Check sheet for the modelled part. Datum: model origin and axes. Units: mm. A direction names the side the tool comes from. Coordinates: 2 decimals unless noted, no trailing zeros. Loops run counter-clockwise (first coordinate to the right, second up) from the corner with the lowest first, then second, coordinate; pieces in that order, holes last.
```python
from build123d import *

# Parameters (mm, degrees)
ESQUISSE1_W             = 105
ESQUISSE1_H             = 30
BOSS_EXTRU_1_DEPTH      = 25
ESQUISSE2_W             = 2
ESQUISSE2_H             = 25
ENL_V_MAT_EXTRU_1_DEPTH = 24
CONG_3_R                = 12
CONG_4_R                = 12
ESQUISSE3_W             = 84
ESQUISSE3_H             = 24
ENL_V_MAT_EXTRU_2_DEPTH = 20
CONG_5_R                = 2
CONG_6_R                = 2
CONG_7_R                = 2


with BuildPart() as part:
    # Esquisse1 → Boss.-Extru.1 (new body)
    with BuildSketch(Plane.XY):
        with Locations((10.65403423, 34.547677262)):
            Rectangle(ESQUISSE1_W, ESQUISSE1_H)
    extrude(amount=BOSS_EXTRU_1_DEPTH)

    # Esquisse2 → Enlèv. mat.-Extru.1 (cut)
    with BuildSketch(Plane.XY.offset(25)):
        with Locations((-34.34596577, 35.047677262)):
            Rectangle(ESQUISSE2_W, ESQUISSE2_H)
        with Locations((55.65403423, 35.047677262)):
            Rectangle(ESQUISSE2_W, ESQUISSE2_H)
    extrude(amount=-ENL_V_MAT_EXTRU_1_DEPTH, mode=Mode.SUBTRACT)

    # Congé3
    cong_3_edges = [part.edges().sort_by_distance(p)[0] for p in [
        (55.65403423, 47.547677262, 1),
        (55.65403423, 22.547677262, 1),
    ]]
    fillet(cong_3_edges, radius=CONG_3_R)

    # Congé4
    cong_4_edges = [part.edges().sort_by_distance(p)[0] for p in [
        (-34.34596577, 47.547677262, 1),
        (-34.34596577, 22.547677262, 1),
    ]]
    fillet(cong_4_edges, radius=CONG_4_R)

    # Esquisse3 → Enlèv. mat.-Extru.2 (cut)
    with BuildSketch(Plane.XY.offset(25)):
        with Locations((10.65403423, 34.547677262)):
            Rectangle(ESQUISSE3_W, ESQUISSE3_H)
    extrude(amount=-ENL_V_MAT_EXTRU_2_DEPTH, mode=Mode.SUBTRACT)

    # Congé5
    cong_5_edges = [part.edges().sort_by_distance(p)[0] for p in [
        (52.65403423, 46.547677262, 15),
        (52.65403423, 22.547677262, 15),
        (-41.84596577, 49.547677262, 12.5),
        (63.15403423, 49.547677262, 12.5),
        (63.15403423, 19.547677262, 12.5),
    ]]
    fillet(cong_5_edges, radius=CONG_5_R)

    # Congé6
    cong_6_edges = [part.edges().sort_by_distance(p)[0] for p in [
        (-31.34596577, 22.547677262, 15),
        (-31.34596577, 46.547677262, 15),
    ]]
    fillet(cong_6_edges, radius=CONG_6_R)

    # Congé7
    cong_7_edges = [part.edges().sort_by_distance(p)[0] for p in [
        (-41.84596577, 19.547677262, 12.5),
    ]]
    fillet(cong_7_edges, radius=CONG_7_R)


solid = part.part
```
1) Section check C-C on y = 32. Enter the section's corners in (x, z), plus the area to 3 significant figures.
Answer sheet:
outline: (-41.85, 0) - (63.15, 0) - (63.15, 25) - (56.65, 25) - (56.65, 1.27) - (54.65, 1.27) - (54.65, 25) - (52.65, 25) - (52.65, 5) - (-31.35, 5) - (-31.35, 25) - (-33.35, 25) - (-33.35, 1.27) - (-35.35, 1.27) - (-35.35, 25) - (-41.85, 25) - close
area: 850 mm2
2) Set-up check for faces 5 (the flat face through (7, 47, 25)), 6 (the cylindrical face through (-30.776, 45.946, 14.86)): record each of +Z, -Z, +X, -X, +Y, -Y from which the full face is reachable in a straight line by a thin tool's end or side.
Answer sheet:
face 5: +Z, +X, -X, +Y, -Y
face 6: +Z
3) Section check D-D on z = 10.75. Enter the section's corners in (x, y), plus the area to 3 significant figures.
Answer sheet:
outline: (-41.85, 21.55) arc R2 ccw to (-39.85, 19.55) - (61.15, 19.55) arc R2 ccw to (63.15, 21.55) - (63.15, 47.55) arc R2 ccw to (61.15, 49.55) - (-39.85, 49.55) arc R2 ccw to (-41.85, 47.55) - close; hole (-35.35, 22.76) - (-33.35, 22.76) - (-33.35, 47.33) - (-35.35, 47.33) - close; hole (-31.35, 24.55) arc R2 ccw to (-29.35, 22.55) - (50.65, 22.55) arc R2 ccw to (52.65, 24.55) - (52.65, 44.55) arc R2 ccw to (50.65, 46.55) - (-29.35, 46.55) arc R2 ccw to (-31.35, 44.55) - close; hole (54.65, 22.76) - (56.65, 22.76) - (56.65, 47.33) - (54.65, 47.33) - close
area: 1,040 mm2
4) Section check A-A on x = 36. Enter the section's corners in (y, z), plus the area to 3 significant figures.
Answer sheet:
outline: (19.55, 0) - (49.55, 0) - (49.55, 25) - (46.55, 25) - (46.55, 5) - (22.55, 5) - (22.55, 25) - (19.55, 25) - close
area: 270 mm2
5) Section check B-B on z = 16.75. Enter the section's corners in (x, y).
Answer sheet:
outline: (-41.85, 21.55) arc R2 ccw to (-39.85, 19.55) - (61.15, 19.55) arc R2 ccw to (63.15, 21.55) - (63.15, 47.55) arc R2 ccw to (61.15, 49.55) - (-39.85, 49.55) arc R2 ccw to (-41.85, 47.55) - close; hole (-35.35, 22.55) - (-33.35, 22.55) - (-33.35, 47.55) - (-35.35, 47.55) - close; hole (-31.35, 24.55) arc R2 ccw to (-29.35, 22.55) - (50.65, 22.55) arc R2 ccw to (52.65, 24.55) - (52.65, 44.55) arc R2 ccw to (50.65, 46.55) - (-29.35, 46.55) arc R2 ccw to (-31.35, 44.55) - close; hole (54.65, 22.55) - (56.65, 22.55) - (56.65, 47.55) - (54.65, 47.55) - close
6) Depth check by flat-ended pin: pin 1 (1.1 mm diameter, centred on x = 56, y = 35, fed in from +Z); pin 2 (7 mm diameter, centred on x = 29.5, y = 34, fed in from +Z). Enter the tip coordinate at first touch or a pass-through.
Answer sheet:
pin 1: stops at z = 1
pin 2: stops at z = 5
7) Mould release check, pull along Y, two halves, no side actions. Record for faces 1 (the flat face through (-35.346, 35, 13)), 2 (the cylindrical face through (55.668, 44.126, 4.609)), 3 (the flat face through (10, 49.548, 12)), 4 (the cylindrical face through (-41.276, 20.149, 12.675)): +Y half, -Y half, draft (parallel to the pull), parting line (faces both ways), or undercut.
Answer sheet:
face 1: undercut
face 2: undercut
face 3: +Y half
face 4: -Y half
8) Scan lines: line 1 (X direction, y = 40.25, z = 3.25); line 2 (X direction, y = 40.75, z = 10.75); line 3 (Y direction, x = 20.5, z = 11.25). Record each from-to range of solid material in increasing order.
Answer sheet:
line 1: x = -41.85 to -35.35, -33.35 to 54.65, 56.65 to 63.15
line 2: x = -41.85 to -35.35, -33.35 to -31.35, 52.65 to 54.65, 56.65 to 63.15
line 3: y = 19.55 to 22.55, 46.55 to 49.55
